Input: part model. Units: mm. Frame: model coordinates. A direction names the side the tool comes from. Give positions to 0.01 mm unless a question says otherwise; leave off trailing zeros. Loops run counter-clockwise (first coordinate to the right, second up) from the corner with the lowest first, then second, coordinate; pieces in that order, holes last.
from build123d import *

# Parameters (mm, degrees)
SKETCH2_R           = 1.5
BOSS_EXTRUDE1_DEPTH = 22
CHAMFER1_SIZE       = 0.3
CUT_EXTRUDE1_DEPTH  = 1.2
SKETCH8_R           = 1.204700538
CUT_EXTRUDE2_DEPTH  = 1
CUT_EXTRUDE2_TAPER  = 45


with BuildPart() as part:
    # Sketch2 → Boss-Extrude1 (new body)
    with BuildSketch(Plane(origin=(0, 0, 0), x_dir=(0, 0, -1), z_dir=(1, 0, 0))):
        Circle(SKETCH2_R)
    extrude(amount=-BOSS_EXTRUDE1_DEPTH)

    # Chamfer1
    chamfer1_edges = [part.edges().sort_by_distance(p)[0] for p in [
        (0, 0, 1.5),
    ]]
    chamfer(chamfer1_edges, length=CHAMFER1_SIZE)

    # Sketch6 → Revolve1 (revolve)
    with BuildSketch(Plane.XY):
        with BuildLine():
            Line((-23.65, 0), (-23.65, 1.5))
            ThreePointArc((-23.65, 1.5), (-23.055944823, 2.284868705), (-22.25, 2.85))
            Line((-22.25, 2.85), (-22, 2.85))
            Line((-22, 2.85), (-22, 0))
            Line((-22, 0), (-23.65, 0))
        make_face()
    revolve(axis=Axis((-22, 0, 0), (1, 0, 0)))

    # Sketch7 → Cut-Extrude1 (cut)
    with BuildSketch(Plane.ZY.offset(23.65)):
        Polygon((0, 1.154700538), (-1, 0.577350269), (-1, -0.577350269), (0, -1.154700538), (1, -0.577350269), (1, 0.577350269), align=None)
    extrude(amount=-CUT_EXTRUDE1_DEPTH, mode=Mode.SUBTRACT)

    # Sketch8 → Cut-Extrude2 (cut)
    with BuildSketch(Plane.ZY.offset(23.65)):
        Circle(SKETCH8_R)
    extrude(amount=-CUT_EXTRUDE2_DEPTH, taper=CUT_EXTRUDE2_TAPER, mode=Mode.SUBTRACT)


solid = part.part
(1) Reachability of faces 5 (the flat face through (0, 0, 0)), 6 (the flat face through (-23.03, 0.87, -0.49)) from +Z, -Z, +X, -X, +Y, -Y: full face, straight path, thin tool, end or side. Return the list, or none.
Values follow:
face 5: +Z, -Z, +X, +Y, -Y
face 6: -X
(2) Cut plane A-A (x = -17). Return the cut outline in (y, z).
Values follow:
outline: circle Ø3 at (0, 0)
(3) Pin query (flat end, axial travel): pin 1 Ø2 at (x, z) = (-5.5, 1) entering from -Y; pin 2 Ø2 at (y, z) = (1, -2) entering from +X; pin 3 Ø3 at (x, z) = (-3.5, -2) entering from +Y. Return the tip coordinate at first contact, or that it passes through.
Values follow:
pin 1: stops at y = -1.5
pin 2: stops at x = -0.04
pin 3: stops at y = 1.41
(4) Cut plane B-B (y = -2.1). Return the cut outline in (x, z), and give its area (3 significant figures).
Values follow:
outline: (-22.25, -1.93) - (-22, -1.93) - (-22, 1.93) - (-22.25, 1.93) arc R2.38 ccw to start
area: 3.62 mm2
(5) Ray query, probe 1 along Y at (x, z) = (-16.25, 0.9); probe 2 along X at (y, z) = (2.5, 0.65); probe 3 along X at (y, z) = (-0.95, -2.05). Return the intervals inside material, ascending.
Values follow:
probe 1: y = -1.2 to 1.2
probe 2: x = -22.7 to -22
probe 3: x = -23.08 to -22
(6) Cut plane C-C (z = -1.9). Return the cut outline in (x, y), and give its area (3 significant figures).
Values follow:
outline: (-22.25, -2.12) - (-22, -2.12) - (-22, 2.12) - (-22.25, 2.12) arc R2.54 ccw to start
area: 4.49 mm2
(7) Mould query, pull axis Z, two halves, no side actions, for faces 1 (the cylindrical face through (-11, 0.07, 1.5)), 2 (the flat face through (-23, 0, -1)), 3 (the flat face through (-22, 1.2, -1.2)), 4 (the flat face through (-23.03, 0.86, 0.51)). Classes: +Z half, -Z half, draft (parallel to the pull), parting line (faces both ways), or undercut.
Values follow:
face 1: parting line
face 2: undercut
face 3: draft
face 4: undercut
